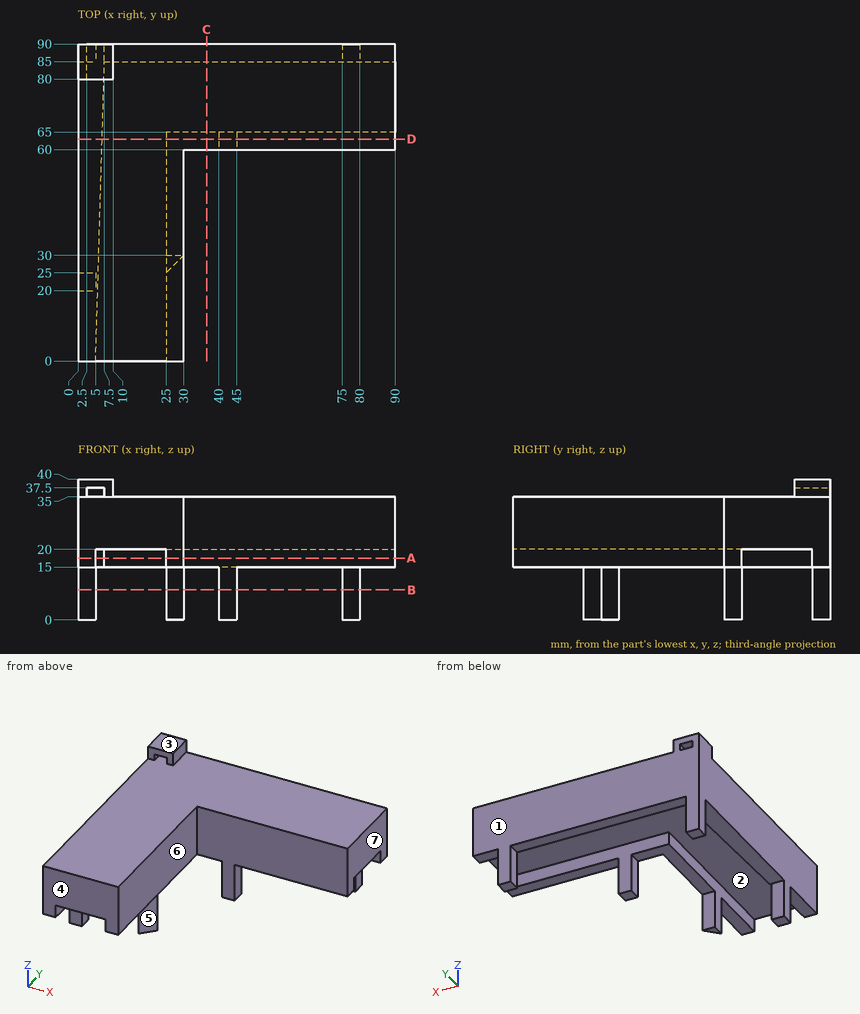
Geometry: see drawing. Coordinates: mm, zero at the bounding-box minimum. A direction names the side the tool comes from. Give positions to 0.01 mm unless a question says otherwise; leave off trailing zeros. Order: outer loops, then holes, each group sorted by start corner. A loop starts at its lowest first (then second) coordinate and runs counter-clockwise, first axis right, second up. Notation, with made-up numbers: M -26,-1.5 L -13,-1.5 A25 cw -13,17.5 Z; hole C 60,-39.5 d4. An arc over 180 degrees is marked long. Answer as CSV lines item,"result". Start each with the question number.
1) Cut plane B-B (z = 8.5). Output: boundary loops of the cut face in (x, y), then the cut area to 4 significant figures.
2) Line query: line 1 (Z direction, x = 67.5, y = 80); line 2 (Z direction, x = 27, y = 7); line 3 (Y direction, x = 70, z = 29). Output: solid intervals per line, ascending. Write a range as from..to.
3) Cut plane A-A (z = 17.5). Output: boundary loops of the cut face in (x, y).
4) First-contact query: P1, Ø3, axis at x = 50.5, z = 35.5, coming from the +Y side; P2, Ø2.5, axis at x = 84.5, y = 87, coming from the -Z side; P3, Ø4, axis at x = 2, z = 9.5, coming from the -Y side; P4, Ø1.5, axis at y = 21.5, z = 35.5, coming from the +X side. Flat tips, straight axial feed; report the tip coordinate or a pass-through.
5) Set-up query: the marked faces 5, 6 and 7. Return all of +Z, -Z, +X, -X, +Y, -Y with unobstructed straight access to the full face (end or side cutting, diameter ignored); none if empty.
6) Mould query, pull axis Y, two halves, no side actions, for the marked faces 1, 2, 3 and 4. Classes: +Y half, -Y half, draft (parallel to the pull), parting line (faces both ways), or undercut.
7) Cut plane C-C (x = 36.5). Output: boundary loops of the cut face in (y, z).
8) Cut plane D-D (y = 63). Output: boundary loops of the cut face in (x, z), then the cut area to 3 significant figures.
Findings below:
1,outline,"M 0,20 L 5,20 L 5,25 L 0,25 Z; M 0,85 L 5,85 L 5,90 L 0,90 Z; M 25,25 L 30,30 L 25,30 Z; M 40,60 L 45,60 L 45,65 L 40,65 Z; M 75,85 L 80,85 L 80,90 L 75,90 Z"
1,area,"112.5 mm²"
2,line 1,"z = 20..35"
2,line 2,"z = 15..35"
2,line 3,"y = 60..90"
3,outline,"M 0,0 L 5,0 L 7.5,85 L 90,85 L 90,90 L 0,90 Z; M 25,0 L 30,0 L 30,60 L 90,60 L 90,65 L 25,65 Z"
4,P1,"stops at y = 90"
4,P2,"stops at z = 15"
4,P3,"stops at y = 20"
4,P4,"stops at x = 30"
5,face 5,"-Z, +X, -Y"
5,face 6,"+Z, -Z, +X, -Y"
5,face 7,"+Z, -Z, +X, +Y, -Y"
6,face 1,"+Y half"
6,face 2,"undercut"
6,face 3,"draft"
6,face 4,"-Y half"
7,outline,"M 60,15 L 65,15 L 65,20 L 85,20 L 85,15 L 90,15 L 90,35 L 60,35 Z"
8,outline,"M 0,15 L 6.85,15 L 6.85,20 L 25,20 L 25,15 L 40,15 L 40,0 L 45,0 L 45,15 L 90,15 L 90,35 L 0,35 Z"
8,area,"1,780 mm²"
